```python
from build123d import *

# Parameters (mm, degrees)
SKETCH1_R           = 2
SKETCH1_R_2         = 1.5
SKETCH1_R_3         = 11.5
SKETCH1_R_4         = 6
BOSS_EXTRUDE1_DEPTH = 3.175
FILLET1_R           = 10
SKETCH2_R           = 2
CUT_EXTRUDE1_DEPTH  = 10
SKETCH3_R           = 2
CUT_EXTRUDE2_DEPTH  = 10
SKETCH4_R           = 1.5
SKETCH4_R_2         = 2
CUT_EXTRUDE3_DEPTH  = 6.35
SKETCH5_R           = 5
CUT_EXTRUDE4_DEPTH  = 3.175


with BuildPart() as part:
    # Sketch1 → Boss-Extrude1 (new body)
    with BuildSketch(Plane(origin=(0, 0, 0), x_dir=(1, 0, 0), z_dir=(0, 1, 0))):
        Polygon((417.700422465, 110), (-26.799577535, 110), (-26.799577535, 0), (417.700422465, 0), (417.700422465, 17.22815868), align=None)
        with Locations(Location((147.450422465, 10, 0), (0, 0, 270))):
            Circle(SKETCH1_R, mode=Mode.SUBTRACT)
        with Locations(Location((103.200422465, 26, 0), (0, 0, 270))):
            Circle(SKETCH1_R_2, mode=Mode.SUBTRACT)
        with Locations(Location((23.200422465, 40, 0), (0, 0, 270))):
            Circle(SKETCH1_R, mode=Mode.SUBTRACT)
        with Locations(Location((89.200422465, 40, 0), (0, 0, 270))):
            Circle(SKETCH1_R_2, mode=Mode.SUBTRACT)
        with Locations(Location((103.200422465, 40, 0), (0, 0, 270))):
            Circle(SKETCH1_R_3, mode=Mode.SUBTRACT)
        with Locations(Location((117.200422465, 40, 0), (0, 0, 270))):
            Circle(SKETCH1_R_2, mode=Mode.SUBTRACT)
        with Locations(Location((177.700422465, 40, 0), (0, 0, 270))):
            Circle(SKETCH1_R_2, mode=Mode.SUBTRACT)
        with Locations(Location((191.700422465, 26, 0), (0, 0, 270))):
            Circle(SKETCH1_R_2, mode=Mode.SUBTRACT)
        with Locations(Location((191.700422465, 40, 0), (0, 0, 270))):
            Circle(SKETCH1_R_3, mode=Mode.SUBTRACT)
        with Locations(Location((205.700422465, 40, 0), (0, 0, 270))):
            Circle(SKETCH1_R_2, mode=Mode.SUBTRACT)
        with Locations(Location((103.200422465, 54, 0), (0, 0, 270))):
            Circle(SKETCH1_R_2, mode=Mode.SUBTRACT)
        with Locations(Location((191.700422465, 54, 0), (0, 0, 270))):
            Circle(SKETCH1_R_2, mode=Mode.SUBTRACT)
        with Locations(Location((282.700422465, 17.22815868, 0), (0, 0, 270))):
            Circle(SKETCH1_R_4, mode=Mode.SUBTRACT)
        with Locations(Location((367.700422465, 40, 0), (0, 0, 270))):
            Circle(SKETCH1_R, mode=Mode.SUBTRACT)
        with Locations(Location((-16.799577535, 85, 0), (0, 0, 270))):
            Circle(SKETCH1_R, mode=Mode.SUBTRACT)
        with Locations(Location((-19.299577535, 102.5, 0), (0, 0, 270))):
            Circle(SKETCH1_R_2, mode=Mode.SUBTRACT)
        with Locations(Location((147.450422465, 85, 0), (0, 0, 270))):
            Circle(SKETCH1_R, mode=Mode.SUBTRACT)
        with Locations(Location((88.075422465, 102.5, 0), (0, 0, 270))):
            Circle(SKETCH1_R_2, mode=Mode.SUBTRACT)
        with Locations(Location((279.700422465, 85, 0), (0, 0, 270))):
            Circle(SKETCH1_R, mode=Mode.SUBTRACT)
        with Locations(Location((195.450422465, 102.5, 0), (0, 0, 270))):
            Circle(SKETCH1_R_2, mode=Mode.SUBTRACT)
        with Locations(Location((302.825422465, 102.5, 0), (0, 0, 270))):
            Circle(SKETCH1_R_2, mode=Mode.SUBTRACT)
        with Locations(Location((407.700422465, 85, 0), (0, 0, 270))):
            Circle(SKETCH1_R, mode=Mode.SUBTRACT)
        with Locations(Location((410.200422465, 102.5, 0), (0, 0, 270))):
            Circle(SKETCH1_R_2, mode=Mode.SUBTRACT)
    extrude(amount=BOSS_EXTRUDE1_DEPTH)

    # Fillet1
    fillet1_edges = [part.edges().sort_by_distance(p)[0] for p in [
        (417.700422465, 1.5875, 0),
        (-26.799577535, 1.5875, 0),
        (-26.799577535, 1.5875, -110),
        (417.700422465, 1.5875, -110),
    ]]
    fillet(fillet1_edges, radius=FILLET1_R)

    # Sketch2 → Cut-Extrude1 (cut)
    with BuildSketch(Plane(origin=(0, 3.175, 0), x_dir=(1, 0, 0), z_dir=(0, 1, 0))):
        with Locations(Location((133.950422465, 55.40559892, 0), (0, 0, 270))):
            Circle(SKETCH2_R)
        with Locations(Location((165.950422465, 55.40559892, 0), (0, 0, 270))):
            Circle(SKETCH2_R)
        with Locations(Location((165.950422465, 23.40559892, 0), (0, 0, 270))):
            Circle(SKETCH2_R)
        with Locations(Location((157.950422465, 47.40559892, 0), (0, 0, 270))):
            Circle(SKETCH2_R)
        with Locations(Location((125.950422465, 47.40559892, 0), (0, 0, 270))):
            Circle(SKETCH2_R)
        with Locations(Location((133.950422465, 23.40559892, 0), (0, 0, 270))):
            Circle(SKETCH2_R)
        with Locations(Location((125.950422465, 31.40559892, 0), (0, 0, 270))):
            Circle(SKETCH2_R)
        with Locations(Location((157.950422465, 31.40559892, 0), (0, 0, 270))):
            Circle(SKETCH2_R)
    extrude(amount=-CUT_EXTRUDE1_DEPTH, mode=Mode.SUBTRACT)

    # Sketch3 → Cut-Extrude2 (cut)
    with BuildSketch(Plane.XZ):
        with Locations(Location((136.950422465, -47.40559892, 0), (0, 0, 270))):
            Circle(SKETCH3_R)
        with Locations(Location((144.950422465, -31.40559892, 0), (0, 0, 270))):
            Circle(SKETCH3_R)
        with Locations(Location((136.950422465, -31.40559892, 0), (0, 0, 270))):
            Circle(SKETCH3_R)
        with Locations(Location((144.950422465, -47.40559892, 0), (0, 0, 270))):
            Circle(SKETCH3_R)
        with Locations(Location((229.950422465, -55.40559892, 0), (0, 0, 270))):
            Circle(SKETCH3_R)
        with Locations(Location((229.950422465, -23.40559892, 0), (0, 0, 270))):
            Circle(SKETCH3_R)
        with Locations(Location((261.950422465, -23.40559892, 0), (0, 0, 270))):
            Circle(SKETCH3_R)
        with Locations(Location((261.950422465, -55.40559892, 0), (0, 0, 270))):
            Circle(SKETCH3_R)
    extrude(amount=-CUT_EXTRUDE2_DEPTH, mode=Mode.SUBTRACT)

    # Sketch4 → Cut-Extrude3 (cut)
    with BuildSketch(Plane(origin=(0, 3.175, 0), x_dir=(1, 0, 0), z_dir=(0, 1, 0))):
        with Locations(Location((21.590660574, 102.5, 0), (0, 0, 270))):
            Circle(SKETCH4_R)
        with Locations(Location((5.664827234, 58.95279946, 0), (0, 0, 270))):
            Circle(SKETCH4_R)
        with Locations(Location((-10.261006106, 15.40559892, 0), (0, 0, 270))):
            Circle(SKETCH4_R)
        with Locations(Location((47.350422465, 50.90559892, 0), (0, 0, 270))):
            Circle(SKETCH4_R_2)
        with Locations(Location((115.670834955, 102.5, 0), (0, 0, 270))):
            Circle(SKETCH4_R)
        with Locations(Location((145.670834955, 102.5, 0), (0, 0, 270))):
            Circle(SKETCH4_R)
        with Locations(Location((175.670834955, 102.5, 0), (0, 0, 270))):
            Circle(SKETCH4_R)
        with Locations(Location((47.350422465, 95.90559892, 0), (0, 0, 270))):
            Circle(SKETCH4_R_2)
        with Locations(Location((21.590660574, 15.40559892, 0), (0, 0, 270))):
            Circle(SKETCH4_R)
        with Locations(Location((47.350422465, 28.40559892, 0), (0, 0, 270))):
            Circle(SKETCH4_R_2)
        with Locations(Location((208.950422465, 80.80559892, 0), (0, 0, 270))):
            Circle(SKETCH4_R_2)
        with Locations(Location((184.950422465, 80.80559892, 0), (0, 0, 270))):
            Circle(SKETCH4_R_2)
        with Locations(Location((109.950422465, 80.80559892, 0), (0, 0, 270))):
            Circle(SKETCH4_R_2)
        with Locations(Location((85.950422465, 80.80559892, 0), (0, 0, 270))):
            Circle(SKETCH4_R_2)
    extrude(amount=-CUT_EXTRUDE3_DEPTH, mode=Mode.SUBTRACT)

    # Sketch5 → Cut-Extrude4 (cut)
    with BuildSketch(Plane(origin=(0, 3.175, 0), x_dir=(1, 0, 0), z_dir=(0, 1, 0))):
        with Locations(Location((47.350422465, 95.90559892, 0), (0, 0, 270))):
            Circle(SKETCH5_R)
        with Locations(Location((47.350422465, 50.90559892, 0), (0, 0, 270))):
            Circle(SKETCH5_R)
        with Locations(Location((47.350422465, 28.40559892, 0), (0, 0, 270))):
            Circle(SKETCH5_R)
    extrude(amount=-CUT_EXTRUDE4_DEPTH, mode=Mode.SUBTRACT)


solid = part.part
```
Work out the finished part from the listing and answer in its coordinate system (mm). Round coordinates to 2 decimals unless told otherwise and drop trailing zeros. One line per question, with ' | ' between items.
Q1. Find section A-A, the plane y = 1.4. State how many separate pieces and enclosed holes the cut face has, then the cut area to 3 significant figures.
Conclusion:
separate pieces: 1 | enclosed holes: 53 | area: 47,100 mm2
Q2. Consider line 1 along Z through (x, y) = (229.5, 2.65); line 2 along X through (y, z) = (0.9, -56); line 3 along Z through (x, y) = (283, 0.85). Determine where each line is inside the solid, lowest interval first. Write a range as from..to.
Conclusion:
line 1: z = -110..-57.35, -53.46..-25.35, -21.46..0 | line 2: x = -26.8..132.04, 135.86..164.04, 167.86..228.04, 231.86..260.04, 263.86..417.7 | line 3: z = -110..-23.22, -11.24..0
Q3. The mould has two halves that part along Z. Classify faces 1 (the cylindrical face through (414.69, 1.61, -107.15)), 2 (the cylindrical face through (44.308, 1.61, -54.873)), 3 (the cylindrical face through (-23.95, 1.61, -3.01)): +Z half, -Z half, draft (parallel to the pull), parting line (faces both ways), or undercut.
Conclusion:
face 1: -Z half | face 2: undercut | face 3: +Z half
